Autodesk Inventor part; units mm, degrees
ref_plane "Work Plane1" through (0, 0, 2.5241) normal (0, 0, 1) x (1, 0, 0)
ref_plane "YZ Plane" through (0, 0, 0) normal (1, 0, 0) x (0, 1, 0)
ref_plane "XZ Plane" through (0, 0, 0) normal (0, 1, 0) x (-1, 0, 0)
ref_plane "Work Plane1" through (0, 0, 2.5241) normal (0, 0, 1) x (1, 0, 0)
sketch "Sketch1" plane through (0, 0, 2.5241) normal (0, 0, 1) x (1, 0, 0)
  line L0 (-4, 272) -> (-4, -8) construction
  line L1 (4, 272) -> (4, -8) construction
  line L2 (76, 272) -> (76, -8) construction
  line L3 (84, 272) -> (84, -8) construction
  line L4 (84, -8) -> (-4, -8) construction
  line L5 (84, 106) -> (80, 106) construction
  line L6 (80, 110) -> (76, 110) construction
  line L7 (-3.365, 272) -> (-3.365, -7.365) construction
  line L8 (-3.365, -7.365) -> (83.365, -7.365) construction
  line L9 (83.365, -7.365) -> (83.365, 272) construction
  line L10 (-3.365, -7.365) -> (83.365, -7.365)
  line L11 (83.365, -7.365) -> (83.365, 107.95)
  line L12 (-3.365, 107.95) -> (-3.365, -7.365)
  circle A0 centre (0, 12) radius 2
  circle A1 centre (80, 12) radius 2
  circle A2 centre (0, 84) radius 2
  circle A3 centre (80, 84) radius 2
  line L13 (21.39, 107.95) -> (21.39, 11.177)
  line L14 (21.39, 11.177) -> (67.11, 11.177)
  line L15 (67.11, 11.177) -> (67.11, 107.95)
  line L16 (83.365, 107.95) -> (67.11, 107.95)
  line L17 (21.39, 107.95) -> (-3.365, 107.95)
  point P0 (0, 0)
  dimension "d0" = 0.635
  dimension "d1" = 8.89
  dimension "d2" = 45.72
  dimension "d18" = 18.542
extrude "Extrusion1" add sketch "Sketch1" along normal blind 10.16
sketch "Sketch2" plane through (0, 0, 12.6841) normal (0, 0, 1) x (1, 0, 0)
  line L0 (83.365, 107.95) -> (67.11, 107.95)
  line L1 (83.365, -7.365) -> (83.365, 107.95)
  line L2 (67.11, 107.95) -> (83.365, 107.95)
  line L3 (83.365, 107.95) -> (83.365, 23.8125)
  line L4 (83.365, 23.8125) -> (67.11, 23.8125)
  line L5 (67.11, 23.8125) -> (67.11, 107.95)
  circle A0 centre (80, 84) radius 2
  circle A1 centre (80, 84) radius 1.9939
  point P0 (0, 0)
  dimension "d5" = 3.9878
extrude "Extrusion2" add sketch "Sketch2" along normal blind 2.54 contours L1 L4 L5 L0
fillet "Fillet1" radius 25.4 1 edges at (75.2375, 107.95, 15.2241)
sketch "Sketch3" plane through (0, 0, 12.6841) normal (0, 0, 1) x (1, 0, 0)
  circle A0 centre (0, 12) radius 2 construction
  circle A1 centre (0, 12) radius 4.8768 construction
  circle A2 centre (0, 84) radius 2 construction
  circle A3 centre (0, 84) radius 4.8768 construction
  circle A4 centre (80, 12) radius 2 construction
  circle A5 centre (80, 12) radius 4.8768 construction
  line L0 (80, 16.8768) -> (84.2234, 14.4384)
  line L1 (84.2234, 14.4384) -> (84.2234, 9.5616)
  line L2 (84.2234, 9.5616) -> (80, 7.1232)
  line L3 (80, 7.1232) -> (75.7766, 9.5616)
  line L4 (75.7766, 9.5616) -> (75.7766, 14.4384)
  line L5 (75.7766, 14.4384) -> (80, 16.8768)
  line L6 (0, 16.8768) -> (4.2234, 14.4384)
  line L7 (4.2234, 14.4384) -> (4.2234, 9.5616)
  line L8 (4.2234, 9.5616) -> (0, 7.1232)
  line L9 (0, 7.1232) -> (-4.2234, 9.5616)
  line L10 (-4.2234, 9.5616) -> (-4.2234, 14.4384)
  line L11 (-4.2234, 14.4384) -> (0, 16.8768)
  line L12 (0, 88.8768) -> (4.2234, 86.4384)
  line L13 (4.2234, 86.4384) -> (4.2234, 81.5616)
  line L14 (4.2234, 81.5616) -> (0, 79.1232)
  line L15 (0, 79.1232) -> (-4.2234, 81.5616)
  line L16 (-4.2234, 81.5616) -> (-4.2234, 86.4384)
  line L17 (-4.2234, 86.4384) -> (0, 88.8768)
  point P0 (0, 0)
  dimension "d9" = 9.7536
  dimension "d10" = 9.7536
  dimension "d11" = 9.7536
extrude "Extrusion3" cut sketch "Sketch3" against normal blind 4.826
sketch "Sketch4" plane through (0, 0, 15.2241) normal (0, 0, 1) x (1, 0, 0)
  circle A0 centre (80, 84) radius 2 construction
  circle A1 centre (80, 84) radius 4.8768 construction
  line L0 (80, 88.8768) -> (84.2234, 86.4384)
  line L1 (84.2234, 86.4384) -> (84.2234, 81.5616)
  line L2 (84.2234, 81.5616) -> (80, 79.1232)
  line L3 (80, 79.1232) -> (75.7766, 81.5616)
  line L4 (75.7766, 81.5616) -> (75.7766, 86.4384)
  line L5 (75.7766, 86.4384) -> (80, 88.8768)
  point P0 (0, 0)
  dimension "d14" = 9.7536
extrude "Extrusion4" cut sketch "Sketch4" against normal blind 4.826
sketch "Sketch5" plane through (0, 0, 12.6841) normal (0, 0, 1) x (1, 0, 0)
  line L0 (-3.365, -7.365) -> (83.365, -7.365)
  line L1 (83.365, -7.365) -> (83.365, 107.95)
  line L2 (-3.365, -7.365) -> (83.365, -7.365)
  line L3 (83.365, -7.365) -> (83.365, 5.335)
  line L4 (83.365, 5.335) -> (-3.365, 5.335)
  line L5 (-3.365, 5.335) -> (-3.365, -7.365)
  point P0 (0, 0)
  dimension "d19" = 12.7
extrude "Extrusion5" cut sketch "Sketch5" against normal blind 5.08
properties part number "Old Back Wall"
Design review of the part built by this model. Coordinates are the model's own, in mm. A direction names the side the tool comes from. Round coordinates to 2 decimals unless told otherwise and drop trailing zeros. Order: outer loops, then holes, each group sorted by start corner. A loop starts at its lowest first (then second) coordinate and runs counter-clockwise, first axis right, second up.
1) Machinability: for faces 1 (the flat face through (75, 23.812, 14)), 2 (the flat face through (21.39, 60, 8)), 3 (the flat face through (77.918, 80.325, 12.845)), which of the approach directions +Z, -Z, +X, -X, +Y, -Y give a long, thin tool a straight path to every point of the face, cutting with its end or side? Answer none if there is none.
The answers:
face 1: +Z, +X, -X, -Y
face 2: +Z, -Z, +Y
face 3: +Z
2) Consider section D-D (y = 50). State the section outline as (x, z) points (3 decimals).
The answers:
outline: (-3.365, 2.524) - (21.39, 2.524) - (21.39, 12.684) - (-3.365, 12.684) - close; (67.11, 2.524) - (83.365, 2.524) - (83.365, 15.224) - (67.11, 15.224) - close
3) Consider section A-A (y = 22). State the section outline as (x, z) points (3 decimals), plus the area to 3 significant figures.
The answers:
outline: (-3.365, 2.524) - (21.39, 2.524) - (21.39, 12.684) - (-3.365, 12.684) - close; (67.11, 2.524) - (83.365, 2.524) - (83.365, 12.684) - (67.11, 12.684) - close
area: 417 mm2
4) Clearance check with flat-ended pins moving along their axes: pin 1 Ø8.5 at (x, y) = (-1.5, 10.5) entering from +Z; pin 2 Ø2.5 at (y, z) = (84, 13.5) entering from +X; pin 3 Ø5 at (x, y) = (0, 84) entering from +Z. State where each tip first meets the part, or that it passes through.
The answers:
pin 1: stops at z = 12.68
pin 2: stops at x = 75.78
pin 3: stops at z = 7.86
5) Consider section C-C (z = 5). State the section outline as (x, y) points (3 decimals), plus the area to 3 significant figures.
The answers:
outline: (-3.365, -7.365) - (83.365, -7.365) - (83.365, 106.321) - (67.11, 106.321) - (67.11, 11.177) - (21.39, 11.177) - (21.39, 107.95) - (-3.365, 107.95) - close; hole circle Ø4 at (0, 12); hole circle Ø4 at (0, 84); hole circle Ø4 at (80, 12); hole circle Ø4 at (80, 84)
area: 5,500 mm2
6) For L1, parallel to X at y = 12, z = 4.25 (3 decimals); L2, parallel to Y at x = 0, z = 6.4 (3 decimals); L3, parallel to X at y = 28, z = 9.75 (3 decimals), list the stretches that pass through material, from the lowest coordinate up.
The answers:
L1: x = -3.365 to -2, 2 to 21.39, 67.11 to 78, 82 to 83.365
L2: y = -7.365 to 10, 14 to 82, 86 to 107.95
L3: x = -3.365 to 21.39, 67.11 to 83.365
7) Draft analysis for pull direction Y (two halves, no side actions). For faces 4 (the flat face through (75, 55, 15.224)), 5 (the flat face through (44, 11.177, 8)), 6 (the flat face through (-1.71, 15.89, 10.3)), 7 (the cylindrical face through (0, 82, 5)), state which applies: released by +Y, released by -Y, zero draft, split by the parting line, or undercut.
The answers:
face 4: zero draft
face 5: released by +Y
face 6: undercut
face 7: undercut
